Autodesk Inventor part; units mm, degrees
ref_plane "YZ Plane" through (0, 0, 0) normal (1, 0, 0) x (0, 1, 0)
ref_plane "XZ Plane" through (0, 0, 0) normal (0, 1, 0) x (-1, 0, 0)
ref_plane "XY Plane" through (0, 0, 0) normal (0, 0, 1) x (1, 0, 0)
sketch "Sketch1" plane through (0, 0, 0) normal (1, 0, 0) x (0, 1, 0)
  line L0 (-21.5, -17.5) -> (21.5, -17.5)
  line L1 (21.5, -17.5) -> (21.5, 1.5)
  line L2 (21.5, 17.5) -> (-21.5, 17.5)
  line L3 (-21.5, 17.5) -> (-21.5, -17.5)
  line L4 (-21.5, -17.5) -> (21.5, 17.5) construction
  line L5 (21.5, -17.5) -> (-21.5, 17.5) construction
  line L6 (18.0188, 17.5) -> (28.5, 17.5)
  line L7 (28.5, 17.5) -> (28.5, 1.5)
  line L8 (28.5, 1.5) -> (21.5, 1.5)
  point P0 (0, 0)
  dimension "d0" = 43
  dimension "d1" = 35
  dimension "d2" = 50
  dimension "d3" = 16
extrude "Extrusion1" add sketch "Sketch1" along normal blind 75
sketch "Sketch2" plane through (0, 28.5, 17.5) normal (0, 1, 0) x (1, 0, 0)
  line L0 (0, 0) -> (75, 0)
  line L1 (65.4712, 0) -> (65.4712, 10)
  line L2 (65.4712, 10) -> (55, 10)
  line L3 (55, 10) -> (55, 11)
  line L4 (55, 11) -> (20, 11)
  line L5 (20, 11) -> (20, 10)
  line L6 (20, 10) -> (10.4712, 10)
  line L7 (10.4712, 10) -> (10.4712, 0)
  line L8 (0, 35) -> (75, 35)
  line L9 (37.5, 35) -> (37.5, 5.3668)
  point P0 (0, 17.5)
  dimension "d6" = 55
  dimension "d7" = 35
  dimension "d8" = 17.5
  dimension "d9" = 11
  dimension "d10" = 10
extrude "Extrusion2" cut sketch "Sketch2" against normal blind 75
sketch "Sketch6" plane through (0, -21.5, 17.5) normal (0, 0, 1) x (1, 0, 0)
  line L0 (0, 50) -> (0, 0)
  line L1 (0, 0) -> (10.4712, 0)
  point P0 (0, 21.5)
  point P1 (5, 7)
  dimension "d31" = 5
  dimension "d32" = 7
hole "Hole1" at (5, -14.5, 17.5) direction (0, 0, -1) diameter 4.134 depth 14.2 tip angle 118
pattern_linear "Rectangular Pattern1" count 2 spacing 36 along (0, 1, 0) count 2 spacing 65 along (1, 0, 0) of "Hole1"
sketch "Sketch8" plane through (0, -21.5, -17.5) normal (0, -1, 0) x (1, 0, 0)
  line L0 (0, 35) -> (0, 0)
  line L1 (0, 35) -> (10.4712, 35)
  point P0 (0, 17.5)
  point P1 (37.5, 11)
  dimension "d55" = 37.5
  dimension "d56" = 24
hole "Hole3" at (37.5, -21.5, -6.5) direction (0, 1, 0) diameter 12 depth 20
sketch "Sketch9" plane through (0, -21.5, -17.5) normal (0, 0, -1) x (-1, 0, 0)
  line L0 (0, 0) -> (0, 43)
  line L1 (0, 0) -> (-75, 0)
  point P0 (0, 21.5)
  point P1 (-34, 7)
  dimension "d64" = 34
  dimension "d65" = 7
hole "Hole4" at (34, -14.5, -17.5) direction (0, 0, 1) diameter 2.459 depth 8.8
sketch "Sketch10" plane through (0, -21.5, -17.5) normal (0, -1, 0) x (1, 0, 0)
  line L0 (0, 35) -> (0, 0)
  line L1 (0, 35) -> (10.4712, 35)
  line L2 (65.4712, 35) -> (75, 35)
  point P0 (0, 17.5)
  point P1 (65, 9)
  point P2 (10, 9)
  dimension "d84" = 10
  dimension "d85" = 55
  dimension "d86" = 26
  dimension "d87" = 26
hole "Hole6" at (65, -21.5, -8.5) at (10, -21.5, -8.5) direction (0, 1, 0) diameter 5.4587 end through all counterbore diameter 11 counterbore depth 7
properties part number "Lose Backe"
Can you work these out from the model? Positions are in its coordinate system, mm. A direction names the side the tool comes from. Coordinates: 2 decimals unless noted, no trailing zeros. Loops run counter-clockwise (first coordinate to the right, second up) from the corner with the lowest first, then second, coordinate; pieces in that order, holes last. Notation, with made-up numbers: (41, -24.75) -> (55, -24.75) arc R29 cw to (55, 9.25) -> close; hole circle Ø6 at (-21.5, -22). An arc over 180 degrees is marked (long way). Answer as a JSON object with one key per item and string values.
1) For P1, Ø9.5, axis at x = 37.5, z = -6.5, coming from the +Y side; P2, Ø3, axis at x = 34, y = -14.5, coming from the +Z side, each with a flat end and sliding along its axis, tell me the tip position at first contact or that it passes through.
Results:
{"P1": "stops at y = 21.5", "P2": "stops at z = 6.5"}
2) Thinking about a two-plate mould opening in Y: for faces 1 (the face through (67.664, 3.752, -7.908)), 2 (the face through (32.78, -14.66, -14.61)), 3 (the face through (37, 28.5, 6)), which applies, pulls with the +Y half, pulls with the -Y half, needs draft (parallel to the pull), parting line crosses it, or undercut?
Results:
{"face 1": "needs draft", "face 2": "undercut", "face 3": "pulls with the +Y half"}
3) Imagine slicing it at B-B (y = 2.5). Please give me the cut outline in (x, z).
Results:
{"outline": "(0, -17.5) -> (75, -17.5) -> (75, 17.5) -> (65.47, 17.5) -> (65.47, 7.5) -> (55, 7.5) -> (55, 6.5) -> (20, 6.5) -> (20, 7.5) -> (10.47, 7.5) -> (10.47, 17.5) -> (0, 17.5) -> close; hole circle Ø5.46 at (10, -8.5); hole circle Ø5.46 at (65, -8.5)"}
4) Imagine slicing it at D-D (z = -8.5). Please give me the cut outline in (x, y).
Results:
{"outline": "(0, -21.5) -> (4.5, -21.5) -> (4.5, -14.5) -> (7.27, -14.5) -> (7.27, 21.5) -> (0, 21.5) -> close; (12.73, -14.5) -> (15.5, -14.5) -> (15.5, -21.5) -> (31.84, -21.5) -> (31.84, -1.5) -> (43.16, -1.5) -> (43.16, -21.5) -> (59.5, -21.5) -> (59.5, -14.5) -> (62.27, -14.5) -> (62.27, 21.5) -> (12.73, 21.5) -> close; (67.73, -14.5) -> (70.5, -14.5) -> (70.5, -21.5) -> (75, -21.5) -> (75, 21.5) -> (67.73, 21.5) -> close"}
5) If I drill on line 1 (X direction, y = -14.5, z = 9.75); line 2 (X direction, y = 10, z = -8.5); line 3 (Y direction, x = 34, z = -12.25), over which ranges is the centre line in solid material (lowest first)?
Results:
{"line 1": "x = 0 to 2.93, 7.07 to 10.47, 65.47 to 67.93, 72.07 to 75", "line 2": "x = 0 to 7.27, 12.73 to 62.27, 67.73 to 75", "line 3": "y = -21.5 to -15.73, -13.27 to 21.5"}
6) For faces 4 (the face through (37, 21.5, -8)), 5 (the face through (4.38, 19.53, 10.3)), 6 (the face through (10.471, 4, 12)), 7 (the face through (14.9, -18, -11)), which set-ups out of +Z, -Z, +X, -X, +Y, -Y let a thin tool reach every point of the face, with its end or its side?
Results:
{"face 4": "-Z, +X, -X, +Y", "face 5": "+Z", "face 6": "+Z, +Y, -Y", "face 7": "-Y"}
7) Imagine slicing it at A-A (z = 13). Please give me the cut outline in (x, y).
Results:
{"outline": "(0, -21.5) -> (10.47, -21.5) -> (10.47, 28.5) -> (0, 28.5) -> close; (65.47, -21.5) -> (75, -21.5) -> (75, 28.5) -> (65.47, 28.5) -> close; hole circle Ø4.13 at (5, -14.5); hole circle Ø4.13 at (5, 21.5); hole circle Ø4.13 at (70, -14.5); hole circle Ø4.13 at (70, 21.5)"}
8) Imagine slicing it at C-C (x = 37.5). Please give me the cut outline in (y, z).
Results:
{"outline": "(-21.5, -17.5) -> (21.5, -17.5) -> (21.5, 1.5) -> (28.5, 1.5) -> (28.5, 6.5) -> (-21.5, 6.5) -> (-21.5, -0.5) -> (-1.5, -0.5) -> (-1.5, -12.5) -> (-21.5, -12.5) -> close"}
